Geometry: final body of the model. Coordinates: model frame, mm. A direction names the side the tool comes from. Give positions to 0.01 mm unless a question says otherwise; leave off trailing zeros. Write each loop counter-clockwise with the first axis right and the second up, starting at its lowest first coordinate (ties: lowest second). Pieces come first, ordered by that corner, then holes. Notation, with made-up numbers: M 57.25,-19 L 94.25,-19 A29 cw 94.25,18 Z; hole C 75,87 d8. An arc over 180 degrees is marked long. Answer as a JSON object with one key per item and string values.
from build123d import *

# Parameters (mm, degrees)
SKETCH1_W           = 14.605
SKETCH1_H           = 33.02
BOSS_EXTRUDE1_DEPTH = 4.572
BOSS_EXTRUDE2_DEPTH = 4.572
BOSS_EXTRUDE3_DEPTH = 11.43
CUT_EXTRUDE1_DEPTH  = 50.300379278
SKETCH5_R           = 1.25000004
SKETCH5_R_2         = 1.25
CUT_EXTRUDE2_DEPTH  = 11.43
SKETCH6_W           = 33.355726526
SKETCH6_H           = 18.831890795
CUT_EXTRUDE3_DEPTH  = 3.175
FILLET1_R           = 1.27


with BuildPart() as part:
    # Sketch1 → Boss-Extrude1 (new body)
    with BuildSketch(Plane.XY):
        with Locations((7.3025, 16.51)):
            Rectangle(SKETCH1_W, SKETCH1_H)
    extrude(amount=BOSS_EXTRUDE1_DEPTH)

    # Sketch2 → Boss-Extrude2 (add)
    with BuildSketch(Plane(origin=(14.605, 0, 0), x_dir=(0, 0, -1), z_dir=(1, 0, 0))):
        Polygon((-4.572, 33.02), (-26.162, 0), (19.05, 0), (0, 33.02), align=None)
    extrude(amount=BOSS_EXTRUDE2_DEPTH)

    # Sketch3 → Boss-Extrude3 (add)
    with BuildSketch(Plane(origin=(19.177, 0, 0), x_dir=(0, 0, -1), z_dir=(1, 0, 0))):
        Polygon((-23.172615385, 4.572), (16.412307692, 4.572), (19.05, 0), (-26.162, 0), align=None)
    extrude(amount=BOSS_EXTRUDE3_DEPTH)

    # Sketch4 → Cut-Extrude1 (cut, through all)
    with BuildSketch(Plane(origin=(0, 4.572, 0), x_dir=(1, 0, 0), z_dir=(0, 1, 0))):
        with BuildLine():
            Line((28.575, 11.224846154), (28.575, 7.414846154))
            ThreePointArc((28.575, 7.414846154), (25.273, 4.112846154), (21.971, 7.414846154))
            Line((21.971, 7.414846154), (21.971, 11.224846154))
            ThreePointArc((21.971, 11.224846154), (25.273, 14.526846154), (28.575, 11.224846154))
        make_face()
        with BuildLine():
            Line((28.575, -14.175153846), (28.575, -17.985153846))
            ThreePointArc((28.575, -17.985153846), (25.273, -21.287153846), (21.971, -17.985153846))
            Line((21.971, -17.985153846), (21.971, -14.175153846))
            ThreePointArc((21.971, -14.175153846), (25.273, -10.873153846), (28.575, -14.175153846))
        make_face()
    extrude(amount=-CUT_EXTRUDE1_DEPTH, mode=Mode.SUBTRACT)

    # Sketch5 → Cut-Extrude2 (cut)
    with BuildSketch(Plane.ZY):
        with Locations((2.286, 26.67)):
            Circle(SKETCH5_R)
        with Locations((2.286, 13.97)):
            Circle(SKETCH5_R_2)
    extrude(amount=-CUT_EXTRUDE2_DEPTH, mode=Mode.SUBTRACT)

    # Sketch6 → Cut-Extrude3 (cut)
    with BuildSketch(Plane(origin=(0, 33.02, 0), x_dir=(1, 0, 0), z_dir=(0, 1, 0))):
        with Locations((16.677863263, -3.376077476)):
            Rectangle(SKETCH6_W, SKETCH6_H)
    extrude(amount=-CUT_EXTRUDE3_DEPTH, mode=Mode.SUBTRACT)

    # Fillet1
    fillet1_edges = [part.edges().sort_by_distance(p)[0] for p in [
        (14.605, 14.9225, 4.572),
        (14.605, 14.9225, 0),
    ]]
    fillet(fillet1_edges, radius=FILLET1_R)


solid = part.part
1) Cut plane B-B on x = 12.5. Return loops of the section in (y, z) (3 decimals).
Geometry check:
{"outline": "M 0,0 L 29.845,0 L 29.845,4.572 L 0,4.572 Z"}
2) Cut plane D-D on y = 13.97. Return loops of the section in (x, z) (3 decimals).
Geometry check:
{"outline": "M 0,0 L 13.335,0 A1.27 cw 14.605,-1.27 L 14.605,-10.99 L 19.177,-10.99 L 19.177,17.028 L 14.605,17.028 L 14.605,5.842 A1.27 cw 13.335,4.572 L 0,4.572 L 0,3.536 L 11.43,3.536 L 11.43,1.036 L 0,1.036 Z"}
3) Cut plane A-A on y = 23.75. Return loops of the section in (x, z) (3 decimals), and give its area (3 significant figures).
Geometry check:
{"outline": "M 0,0 L 13.335,0 A1.27 cw 14.605,-1.27 L 14.605,-5.348 L 19.177,-5.348 L 19.177,10.633 L 14.605,10.633 L 14.605,5.842 A1.27 cw 13.335,4.572 L 0,4.572 Z", "area": "141 mm2"}
4) Pull-direction query (Z, two-part tool) for faces 4 (the flat face through (0, 15, 1)), 5 (the flat face through (7, 15, 4.572)), 6 (the flat face through (28.575, 2, 16)); classes: pulls with the +Z half, pulls with the -Z half, needs draft (parallel to the pull), parting line crosses it, or undercut.
Geometry check:
{"face 4": "needs draft", "face 5": "pulls with the +Z half", "face 6": "undercut"}
5) Cut plane C-C on y = 19.5. Return loops of the section in (x, z) (3 decimals), and give its area (3 significant figures).
Geometry check:
{"outline": "M 0,0 L 13.335,0 A1.27 cw 14.605,-1.27 L 14.605,-7.8 L 19.177,-7.8 L 19.177,13.412 L 14.605,13.412 L 14.605,5.842 A1.27 cw 13.335,4.572 L 0,4.572 Z", "area": "164 mm2"}
6) Line query: line 1 (Z direction, x = 23, y = 1.75); line 2 (X direction, y = 4.5, z = -10.5) (3 decimals); line 3 (Y direction, x = 22.5, z = -4). Output: solid intervals per line, ascending. Write a range as from..to.
Geometry check:
{"line 1": "z = -18.04..-13.62, -5.02..11.78, 20.38..25.02", "line 2": "x = 14.605..21.971, 28.575..30.607", "line 3": "y = 0..4.57"}
7) Set-up query: faces 1 (the cylindrical face through (5.63, 25.45, 2.02)), 2 (the flat face through (28.575, 2, -9)), 3 (the flat face through (19.177, 15, 4)). Return all of +Z, -Z, +X, -X, +Y, -Y with unobstructed straight access to the full face (end or side cutting, diameter ignored); none if empty.
Geometry check:
{"face 1": "-X", "face 2": "+Y, -Y", "face 3": "+Z, -Z, +X, +Y"}
8) Contact query for flat-ended pins moving along their axis: P1, Ø5, axis at x = 16.5, y = 11.5, coming from the -Z side; P2, Ø4, axis at y = 26.67, z = 2.286, coming from the +X side; P3, Ø10, axis at y = 12.5, z = 14, coming from the -X side (3 decimals); P4, Ø8, axis at x = 7.5, z = 3.5, coming from the -Y side. Output: stop coordinate, or through.
Geometry check:
{"P1": "stops at z = -13.86", "P2": "stops at x = 19.18", "P3": "stops at x = 14.605", "P4": "stops at y = 0"}
